Could you check a few things on this model? Use its own coordinates, in mm. Face numbers are marked on the shaded views. A direction names the side the tool comes from. Coordinates: 2 decimals unless noted, no trailing zeros. Order: outer loops, then holes, each group sorted by start corner. A loop starts at its lowest first (then second) coordinate and runs counter-clockwise, first axis right, second up. Notation, with made-up numbers: (-32.5, 88) - (8.5, 88) arc R37 ccw to (8.5, 127) - close; hole circle Ø11 at (-31.75, 28.5). An arc over 180 degrees is marked (long way). One line per item, written item: value.
from build123d import *

# Parameters (mm, degrees)
SKETCH1_R           = 75
BOSS_EXTRUDE1_DEPTH = 20
SKETCH2_R           = 10
SKETCH2_R_2         = 7.5
BOSS_EXTRUDE2_DEPTH = 9
SKETCH3_R           = 7.5
CUT_EXTRUDE1_DEPTH  = 20
SKETCH4_R           = 15.621868033
CUT_EXTRUDE2_DEPTH  = 60


with BuildPart() as part:
    # Sketch1 → Boss-Extrude1 (new body)
    with BuildSketch(Plane(origin=(0, 0, 0), x_dir=(1, 0, 0), z_dir=(0, 1, 0))):
        Circle(SKETCH1_R)
    extrude(amount=BOSS_EXTRUDE1_DEPTH)

    # Sketch2 → Boss-Extrude2 (add)
    with BuildSketch(Plane(origin=(0, 20, 0), x_dir=(1, 0, 0), z_dir=(0, 1, 0))):
        with Locations((-50, 0)):
            Circle(SKETCH2_R)
        with Locations((-50, 0)):
            Circle(SKETCH2_R_2, mode=Mode.SUBTRACT)
        with Locations((-31.174490093, 39.091574123)):
            Circle(SKETCH2_R)
        with Locations((-31.174490093, 39.091574123)):
            Circle(SKETCH2_R_2, mode=Mode.SUBTRACT)
        with Locations((11.126046698, 48.746395609)):
            Circle(SKETCH2_R)
        with Locations((11.126046698, 48.746395609)):
            Circle(SKETCH2_R_2, mode=Mode.SUBTRACT)
        with Locations((45.048443395, 21.694186956)):
            Circle(SKETCH2_R)
        with Locations((45.048443395, 21.694186956)):
            Circle(SKETCH2_R_2, mode=Mode.SUBTRACT)
        with Locations((45.048443395, -21.694186956)):
            Circle(SKETCH2_R)
        with Locations((45.048443395, -21.694186956)):
            Circle(SKETCH2_R_2, mode=Mode.SUBTRACT)
        with Locations((11.126046698, -48.746395609)):
            Circle(SKETCH2_R)
        with Locations((11.126046698, -48.746395609)):
            Circle(SKETCH2_R_2, mode=Mode.SUBTRACT)
        with Locations((-31.174490093, -39.091574123)):
            Circle(SKETCH2_R)
        with Locations((-31.174490093, -39.091574123)):
            Circle(SKETCH2_R_2, mode=Mode.SUBTRACT)
    extrude(amount=BOSS_EXTRUDE2_DEPTH)

    # Sketch3 → Cut-Extrude1 (cut)
    with BuildSketch(Plane(origin=(0, 20, 0), x_dir=(1, 0, 0), z_dir=(0, 1, 0))):
        Circle(SKETCH3_R)
        with BuildLine():
            Line((-96.640436965, 20), (-45, 20))
            ThreePointArc((-45, 20), (-25, 0), (-45, -20))
            Line((-45, -20), (-96.640436965, -20))
            Line((-96.640436965, -20), (-96.640436965, 20))
        make_face()
    extrude(amount=-CUT_EXTRUDE1_DEPTH, mode=Mode.SUBTRACT)

    # Sketch4 → Cut-Extrude2 (cut)
    with BuildSketch(Plane(origin=(0, 0, 0), x_dir=(1, 0, 0), z_dir=(0, 1, 0))):
        with Locations((-50, 0)):
            Circle(SKETCH4_R)
    extrude(amount=CUT_EXTRUDE2_DEPTH, mode=Mode.SUBTRACT)


solid = part.part
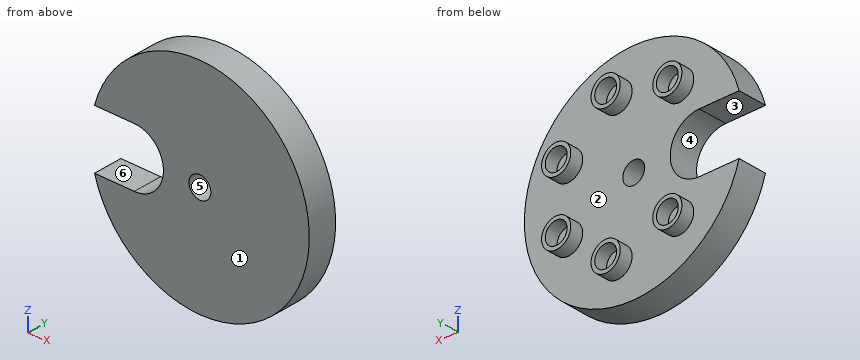
Item 1: I'm going to push flat-ended pins straight in: pin 1 Ø3 at (y, z) = (16.5, -40) entering from -X; pin 2 Ø9 at (x, z) = (-31.17, -39.09) entering from +Y; pin 3 Ø6 at (x, y) = (44, 10.5) entering from -Z. Where does each tip first touch, or does it pass through?
Conclusion:
pin 1: x = -64.36
pin 2: y = 20
pin 3: z = -62.8
Item 2: Thinking about a two-plate mould opening in X: for the marked faces 4, 5 and 6, which applies, pulls with the +X half, pulls with the -X half, needs draft (parallel to the pull), parting line crosses it, or undercut?
Conclusion:
face 4: pulls with the -X half
face 5: undercut
face 6: needs draft
Item 3: I want a section at C-C on y = 22.75. Give the number of separate pieces and of enclosed holes in the cut face, then the cut area to 3 significant figures.
Conclusion:
separate pieces: 6
enclosed holes: 6
area: 825 mm²
Item 4: For the marked faces 1, 2 and 3, which set-ups out of +Z, -Z, +X, -X, +Y, -Y let a thin tool reach every point of the face, with its end or its side?
Conclusion:
face 1: +Z, -Z, +X, -X, -Y
face 2: +Y
face 3: -X, +Y, -Y
Item 5: If I drill on probe 1 along Z at (x, y) = (-30.5, 27.25); probe 2 along Z at (x, y) = (39, 23); probe 3 along X at (y, z) = (4.75, 0), over which ranges is the centre line in solid material (lowest first)?
Conclusion:
probe 1: -49.07 to -46.56, -31.62 to -29.11, 29.11 to 31.62, 46.56 to 49.07
probe 2: -29.66 to -26.13, -17.26 to -13.73, 13.73 to 17.26, 26.13 to 29.66
probe 3: -25 to -7.5, 7.5 to 75
Item 6: I want a section at A-A on x = -54.5. Please give me the cut outline in (y, z).
Conclusion:
outline: (0, -51.52) - (20, -51.52) - (20, -20) - (0, -20) - close; (0, 20) - (20, 20) - (20, 51.52) - (0, 51.52) - close
Item 7: I want a section at B-B on z = 0. Please give me the cut outline in (x, y).
Conclusion:
outline: (-25, 0) - (-7.5, 0) - (-7.5, 20) - (-25, 20) - close; (7.5, 0) - (75, 0) - (75, 20) - (7.5, 20) - close
Item 8: I want a section at D-D on x = 60. Please give me the cut outline in (y, z), then the cut area to 3 significant figures.
Conclusion:
outline: (0, -45) - (20, -45) - (20, 45) - (0, 45) - close
area: 1,800 mm²
